from build123d import *

# Parameters (mm, degrees)
SKETCH_1_W          = 71.5
SKETCH_1_H          = 25.7
EXTRUDE_1_DEPTH     = 7.5
CUT_EXTRUDE_1_DEPTH = 0.3


with BuildPart() as part:
    # 草图1 → 凸台-拉伸1 (new body)
    with BuildSketch(Plane(origin=(0, 0, 0), x_dir=(1, 0, 0), z_dir=(0, 1, 0))):
        with Locations((35.75, -12.85)):
            Rectangle(SKETCH_1_W, SKETCH_1_H)
    extrude(amount=EXTRUDE_1_DEPTH)

    # 草图2 → 切除-拉伸1 (cut)
    with BuildSketch(Plane.XZ):
        Polygon((69.025126266, 25.7), (2.474873734, 25.7), (0, 23.225126266), (0, 2.474873734), (2.474873734, 0), (69.025126266, 0), (71.5, 2.474873734), (71.5, 23.225126266), align=None)
    extrude(amount=-CUT_EXTRUDE_1_DEPTH, mode=Mode.SUBTRACT)


solid = part.part
Design review of the part built by this model. Coordinates are the model's own, in mm. Round coordinates to 2 decimals unless told otherwise and drop trailing zeros. Loops run counter-clockwise (first coordinate to the right, second up) from the corner with the lowest first, then second, coordinate; pieces in that order, holes last. Notation, with made-up numbers: (18, 64.25) - (66, 64.25) arc R25 ccw to (66, 79.25) - close; hole circle Ø7 at (89.25, 20). An arc over 180 degrees is marked (long way). One line per item, written item: value. Start each with the question number.
1) Consider section A-A on x = 38.5. Give the boundary of the cut face in (y, z).
2) To check wall thickness, follow L1, parallel to Y at x = 37.5, z = 10. State the ranges of the line that lie inside material, in increasing order. Write a range as from..to.
3) Consider section B-B on z = 21.5. Give the boundary of the cut face in (x, y), then the cut area to 3 significant figures.
4) Insertion check: pin 1 Ø8 at (x, z) = (22.5, 19) entering from -Y. The pin has a flat end and moves straight along its axis. Give the tip position at first contact, or say it passes through.
Reported:
1. outline: (0.3, 0) - (7.5, 0) - (7.5, 25.7) - (0.3, 25.7) - close
2. L1: y = 0.3..7.5
3. outline: (0, 0.3) - (71.5, 0.3) - (71.5, 7.5) - (0, 7.5) - close
3. area: 515 mm^2
4. pin 1: stops at y = 0.3
